Source: CAD feature listing. Evaluate the final solid. Frame: model axes, mm. Face numbers are marked on the shaded views. Give positions to 0.01 mm unless a question says otherwise; leave off trailing zeros. Write each loop counter-clockwise with the first axis right and the second up, starting at its lowest first coordinate (ties: lowest second). Pieces come first, ordered by that corner, then holes. Notation, with made-up numbers: (30, -23.5) - (80, -23.5) arc R5 cw to (80, -18.5) - close; hole circle Ø2 at (71, 25). An arc over 180 degrees is marked (long way). Answer as a JSON object with one key per item and string values. Group by question number.
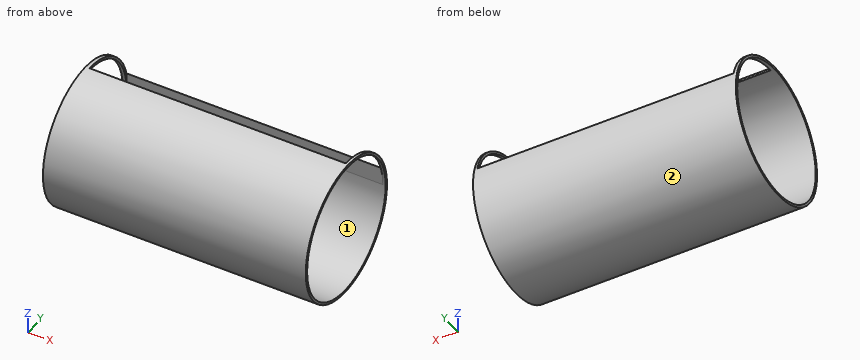
from build123d import *

# Parameters (mm, degrees)
F0_R     = 76.311226
F1_DEPTH = 287.02
F2_R     = 73.720997
F3_DEPTH = 1714.5
F4_W     = 279.827215
F4_H     = 69.845937
F5_DEPTH = 122.428


with BuildPart() as f1:
    # F0 (on Right) → F1 (new body)
    with BuildSketch(Plane.YZ):
        Circle(F0_R)
    extrude(amount=-F1_DEPTH)

    # F2 (on Right) → F3 (cut)
    with BuildSketch(Plane.YZ):
        Circle(F2_R)
    extrude(amount=-F3_DEPTH, mode=Mode.SUBTRACT)

    # F4 (on Top) → F5 (cut)
    with BuildSketch(Plane.XY):
        with Locations((-142.993759, 38.803298)):
            Rectangle(F4_W, F4_H)
    extrude(amount=F5_DEPTH, mode=Mode.SUBTRACT)


solid = f1.part
Q1. First-contact query: pin 1 Ø8 at (x, z) = (-133, -58) entering from -Y; pin 2 Ø4 at (x, z) = (-175.5, 34.5) entering from +Y; pin 3 Ø3 at (x, z) = (-90.5, -24.5) entering from -Y. Flat tips, straight axial feed; report the tip coordinate or a pass-through.
Q2. Section A-A on y = 0. Return the cut outline in (x, z), then the cut area to 3 significant figures.
Q3. Ray query, probe 1 along Y at (x, z) = (-223, -3); probe 2 along Z at (x, y) = (-94, 0); probe 3 along Y at (x, z) = (-152.5, -35.5). Return the intervals inside material, ascending. Write a range as [from, to].
Q4. Section D-D on y = -51. Return the cut outline in (x, z), then the cut area to 3 significant figures.
Q5. Section B-B on z = 5. Return the cut outline in (x, y).
Q6. Draft query along Z for the marked faces 1 and 2. Return one class per face: released by +Z, released by -Z, zero draft, split by the parting line, or undercut.
Taken from the geometry:
{
 "1": {"pin 1": "stops at y = -53.92", "pin 2": "stops at y = -64.05", "pin 3": "stops at y = -72.76"},
 "2": {"outline": "(-287.02, -76.31) - (0, -76.31) - (0, -73.72) - (-287.02, -73.72) - close; (-287.02, 73.72) - (0, 73.72) - (0, 76.31) - (-287.02, 76.31) - close", "area": "1,490 mm²"},
 "3": {"probe 1": "y = [-76.25, -73.66], [73.66, 76.25]", "probe 2": "z = [-76.31, -73.72], [73.72, 76.31]", "probe 3": "y = [-67.55, -64.61], [64.61, 67.55]"},
 "4": {"outline": "(-287.02, -56.77) - (0, -56.77) - (0, -53.23) - (-287.02, -53.23) - close; (-287.02, 53.23) - (0, 53.23) - (0, 56.77) - (-287.02, 56.77) - close", "area": "2,030 mm²"},
 "5": {"outline": "(-287.02, -76.15) - (0, -76.15) - (0, -73.55) - (-287.02, -73.55) - close; (-287.02, 73.55) - (-282.91, 73.55) - (-282.91, 73.73) - (-3.08, 73.73) - (-3.08, 73.55) - (0, 73.55) - (0, 76.15) - (-287.02, 76.15) - close"},
 "6": {"face 1": "undercut", "face 2": "split by the parting line"}
}
